from build123d import *

# Parameters (mm, degrees)
BOSS_EXTRUDE1_DEPTH = 60
SKETCH2_R           = 1.5
CUT_EXTRUDE1_DEPTH  = 10
SKETCH3_R           = 1.5
CUT_EXTRUDE2_DEPTH  = 10


with BuildPart() as part:
    # Sketch1 → Boss-Extrude1 (new body)
    with BuildSketch(Plane(origin=(0, 0, 0), x_dir=(0, 0, -1), z_dir=(1, 0, 0))):
        Polygon((0, 0), (0, 22), (2, 22), (2, 2), (17, 2), (17, 0), align=None)
    extrude(amount=BOSS_EXTRUDE1_DEPTH)

    # Sketch2 → Cut-Extrude1 (cut)
    with BuildSketch(Plane.XZ):
        with Locations(Location((30, -8.5, 0), (0, 0, 270))):
            Circle(SKETCH2_R)
        with Locations(Location((12, -8.5, 0), (0, 0, 270))):
            Circle(SKETCH2_R)
        with Locations(Location((48, -8.5, 0), (0, 0, 270))):
            Circle(SKETCH2_R)
    extrude(amount=-CUT_EXTRUDE1_DEPTH, mode=Mode.SUBTRACT)

    # Sketch3 → Cut-Extrude2 (cut)
    with BuildSketch(Plane.XY):
        with Locations((30, 10)):
            Circle(SKETCH3_R)
        with Locations((12, 10)):
            Circle(SKETCH3_R)
        with Locations((48, 10)):
            Circle(SKETCH3_R)
    extrude(amount=-CUT_EXTRUDE2_DEPTH, mode=Mode.SUBTRACT)


solid = part.part
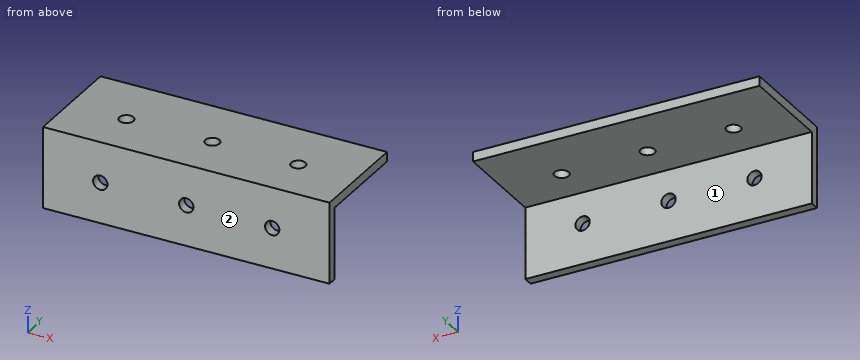
Can you work these out from the model? Positions are in its coordinate system, mm. Face numbers are marked on the shaded views. A direction names the side the tool comes from. Round coordinates to 2 decimals unless told otherwise and drop trailing zeros. Order: outer loops, then holes, each group sorted by start corner. A loop starts at its lowest first (then second) coordinate and runs counter-clockwise, first axis right, second up. Notation, with made-up numbers: (3.5, 73) - (39.5, 73) arc R11 cw to (39.5, 86) - close; hole circle Ø4 at (24.5, -36). An arc over 180 degrees is marked (long way). Answer in a Markdown table with one row per item.
(1) For P1, Ø4, axis at x = 12, y = 10, coming from the -Z side; P2, Ø1, axis at x = 24, z = -3.5, coming from the +Y side, each with a flat end and sliding along its axis, tell me the tip position at first contact or that it passes through.
From the geometry:
| item | result |
|---|---|
| P1 | stops at z = -2 |
| P2 | stops at y = 2 |
(2) Suppose I cut it at C-C, the plane x = 45.5. Please give me the cut outline in (y, z).
From the geometry:
| item | result |
|---|---|
| outline | (0, -17) - (2, -17) - (2, -2) - (22, -2) - (22, 0) - (0, 0) - close |
(3) Please list where these lines run through material, in increasing order: L1, parallel to X at y = 0.75, z = -8.5; L2, parallel to Y at x = 30, z = -1.05; L3, parallel to Z at x = 23, y = 18.25. Write a range as from..to.
From the geometry:
| item | result |
|---|---|
| L1 | x = 0..10.5, 13.5..28.5, 31.5..46.5, 49.5..60 |
| L2 | y = 0..8.5, 11.5..22 |
| L3 | z = -2..0 |
(4) Suppose I cut it at B-B, the plane y = 10. Please give me the cut outline in (x, z), plus the area to 3 significant figures.
From the geometry:
| item | result |
|---|---|
| outline | (0, -2) - (10.5, -2) - (10.5, 0) - (0, 0) - close; (13.5, -2) - (28.5, -2) - (28.5, 0) - (13.5, 0) - close; (31.5, -2) - (46.5, -2) - (46.5, 0) - (31.5, 0) - close; (49.5, -2) - (60, -2) - (60, 0) - (49.5, 0) - close |
| area | 102 mm2 |
(5) Suppose I cut it at A-A, the plane x = 12. Please give me the cut outline in (y, z), plus the area to 3 significant figures.
From the geometry:
| item | result |
|---|---|
| outline | (0, -17) - (2, -17) - (2, -10) - (0, -10) - close; (0, -7) - (2, -7) - (2, -2) - (8.5, -2) - (8.5, 0) - (0, 0) - close; (11.5, -2) - (22, -2) - (22, 0) - (11.5, 0) - close |
| area | 62.0 mm2 |
(6) Suppose I cut it at D-D, the plane z = -3. Please give me the cut outline in (x, y).
From the geometry:
| item | result |
|---|---|
| outline | (0, 0) - (60, 0) - (60, 2) - (0, 2) - close |
(7) Which directions (+Z, -Z, +X, -X, +Y, -Y) give clear straight access to the entire face, cutting with the end or side of a thin tool? Please do the marked faces 1 and 2.
From the geometry:
| item | result |
|---|---|
| face 1 | -Z, +X, -X, +Y |
| face 2 | +Z, -Z, +X, -X, -Y |
